Can you work these out from the model? Positions are in its coordinate system, mm. Face numbers are marked on the shaded views. A direction names the side the tool comes from. Give positions to 0.01 mm unless a question says otherwise; leave off trailing zeros. Order: outer loops, then holes, each group sorted by start corner. A loop starts at its lowest first (then second) coordinate and runs counter-clockwise, first axis right, second up. Notation, with made-up numbers: (13.25, 28) - (38.25, 28) arc R16 cw to (38.25, 47) - close; hole circle Ø7 at (76, 35.25). An arc over 180 degrees is marked (long way). Return JSON: item names as keys, results as strings.
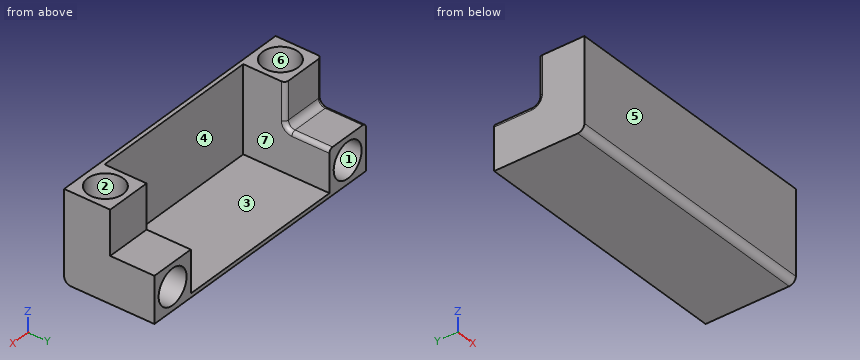
```python
from build123d import *

# Parameters (mm, degrees)
SKETCH1_R           = 13.2
BOSS_EXTRUDE3_DEPTH = 5
SKETCH1_6_W         = 100
SKETCH1_6_H         = 55
SKETCH1_6_R         = 13.2
BOSS_EXTRUDE4_DEPTH = 55
SKETCH2_W           = 65.6
SKETCH2_H           = 52
CUT_EXTRUDE1_DEPTH  = 52
SKETCH3_R           = 13.2
CUT_EXTRUDE2_DEPTH  = 22.6
SKETCH4_W           = 20.6
SKETCH4_H           = 20.6
CUT_EXTRUDE4_DEPTH  = 39
SKETCH9_R           = 13.2
BOSS_EXTRUDE5_DEPTH = 12.4
BOSS_EXTRUDE7_START = 12.4
SKETCH10_R          = 13.2
BOSS_EXTRUDE7_DEPTH = 12.4
MIRROR1_START       = 30.398461356
MIRROR1_OUTLINE_R   = 13.2
MIRROR1_DEPTH       = 37.001538644
MIRROR1_2_OUTLINE_W = 100
MIRROR1_2_OUTLINE_H = 67.4
MIRROR1_2_OUTLINE_R = 13.2
MIRROR1_2_DEPTH     = 3
MIRROR1_3_OUTLINE_W = 34.4
MIRROR1_3_OUTLINE_H = 33
MIRROR1_3_DEPTH     = 4.001538644
MIRROR1_START_2     = 3
MIRROR1_4_OUTLINE_R = 13.2
MIRROR1_4_DEPTH     = 0.998461256
MIRROR1_START_3     = 3.998461256
MIRROR1_5_OUTLINE_R = 13.2
MIRROR1_5_DEPTH     = 26.4000001
MIRROR1_START_4     = 4.9
MIRROR1_6_OUTLINE_R = 13.2
MIRROR1_6_DEPTH     = 35
FILLET3_R           = 5
FILLET4_R           = 5
FILLET5_R           = 3
FILLET6_R           = 3


with BuildPart() as part:
    # Sketch1 → Boss-Extrude3 (new body)
    with BuildSketch(Plane(origin=(0, 0, 0), x_dir=(1, 0, 0), z_dir=(0, 1, 0))):
        with Locations(Location((-32.8, 10.3, 0), (0, 0, 270))):
            Circle(SKETCH1_R)
    boss_extrude3 = extrude(amount=BOSS_EXTRUDE3_DEPTH)

    # Sketch1<6> → Boss-Extrude4 (add)
    with BuildSketch(Plane(origin=(0, 0, 0), x_dir=(1, 0, 0), z_dir=(0, 1, 0))):
        Rectangle(SKETCH1_6_W, SKETCH1_6_H)
        with Locations(Location((-32.8, 10.3, 0), (0, 0, 270))):
            Circle(SKETCH1_6_R, mode=Mode.SUBTRACT)
    extrude(amount=BOSS_EXTRUDE4_DEPTH)

    # Sketch2 → Cut-Extrude1 (cut)
    with BuildSketch(Plane(origin=(0, 55, 0), x_dir=(1, 0, 0), z_dir=(0, 1, 0))):
        with Locations((17.2, -1.5)):
            Rectangle(SKETCH2_W, SKETCH2_H)
    extrude(amount=-CUT_EXTRUDE1_DEPTH, mode=Mode.SUBTRACT)

    # Sketch3 → Cut-Extrude2 (cut)
    with BuildSketch(Plane.XY.offset(27.5)):
        with Locations((-32.801538644, 17.198461356)):
            Circle(SKETCH3_R)
    extrude(amount=-CUT_EXTRUDE2_DEPTH, mode=Mode.SUBTRACT)

    # Sketch4 → Cut-Extrude4 (cut)
    with BuildSketch(Plane.ZY.offset(50)):
        with Locations((17.2, 44.7)):
            Rectangle(SKETCH4_W, SKETCH4_H)
    extrude(amount=-CUT_EXTRUDE4_DEPTH, mode=Mode.SUBTRACT)

    # Sketch9 → Boss-Extrude5 (add)
    with BuildSketch(Plane(origin=(0, 55, 0), x_dir=(1, 0, 0), z_dir=(0, 1, 0))):
        Polygon((-50, -6.9), (-15.6, -6.9), (-15.6, 24.5), (50, 24.5), (50, 27.5), (-50, 27.5), align=None)
        with Locations(Location((-32.8, 10.3, 0), (0, 0, 270))):
            Circle(SKETCH9_R, mode=Mode.SUBTRACT)
    extrude(amount=BOSS_EXTRUDE5_DEPTH)

    # Sketch10 → Boss-Extrude7 (add)
    with BuildSketch(Plane.XY.offset(27.5).offset(BOSS_EXTRUDE7_START)):
        Polygon((-15.6, 3), (-15.6, 34.4), (-50, 34.4), (-50, 0), (50, 0), (50, 3), align=None)
        with Locations((-32.801538644, 17.198461356)):
            Circle(SKETCH10_R, mode=Mode.SUBTRACT)
    extrude(amount=-BOSS_EXTRUDE7_DEPTH)

    # Mirror1: read off the stored shape, not the designer's step
    # Mirror1 outline → Mirror1 (add)
    with BuildSketch(Plane(origin=(0, 0, 0), x_dir=(1, 0, 0), z_dir=(0, 1, 0)).offset(MIRROR1_START)):
        Polygon((150, -6.9), (150, 27.5), (50, 27.5), (50, 24.5), (115.6, 24.5), (115.6, -6.9), align=None)
        with Locations((132.8, 10.3)):
            Circle(MIRROR1_OUTLINE_R, mode=Mode.SUBTRACT)
    extrude(amount=MIRROR1_DEPTH)

    # Mirror1 2 outline → Mirror1 2 (add)
    with BuildSketch(Plane(origin=(0, 0, 0), x_dir=(1, 0, 0), z_dir=(0, 1, 0))):
        with Locations((100, -6.2)):
            Rectangle(MIRROR1_2_OUTLINE_W, MIRROR1_2_OUTLINE_H)
        with Locations((132.8, 10.3)):
            Circle(MIRROR1_2_OUTLINE_R, mode=Mode.SUBTRACT)
    extrude(amount=MIRROR1_2_DEPTH)

    # Mirror1 3 outline → Mirror1 3 (add)
    with BuildSketch(Plane(origin=(0, 0, 0), x_dir=(1, 0, 0), z_dir=(0, 1, 0)).offset(MIRROR1_START)):
        with Locations((132.8, -23.4)):
            Rectangle(MIRROR1_3_OUTLINE_W, MIRROR1_3_OUTLINE_H)
    extrude(amount=MIRROR1_3_DEPTH)

    # Mirror1 4 outline → Mirror1 4 (add)
    with BuildSketch(Plane(origin=(0, 0, 0), x_dir=(1, 0, 0), z_dir=(0, 1, 0)).offset(MIRROR1_START_2)):
        Polygon((150, 27.5), (50, 27.5), (50, 24.5), (115.6, 24.5), (115.6, -39.9), (150, -39.9), align=None)
        with Locations((132.8, 10.3)):
            Circle(MIRROR1_4_OUTLINE_R, mode=Mode.SUBTRACT)
    extrude(amount=MIRROR1_4_DEPTH)

    # Mirror1 5 outline → Mirror1 5 (add)
    with BuildSketch(Plane(origin=(0, 0, 0), x_dir=(1, 0, 0), z_dir=(0, 1, 0)).offset(MIRROR1_START_3)):
        Polygon((150, -39.9), (150, 27.5), (50, 27.5), (50, 24.5), (115.6, 24.5), (115.6, -39.9), align=None)
        with Locations((132.8, 10.3)):
            Circle(MIRROR1_5_OUTLINE_R, mode=Mode.SUBTRACT)
    extrude(amount=MIRROR1_5_DEPTH)

    # Mirror1 6 outline → Mirror1 6 (cut)
    with BuildSketch(Plane.XY.offset(MIRROR1_START_4)):
        with Locations((132.801538644, 17.198461356)):
            Circle(MIRROR1_6_OUTLINE_R)
    extrude(amount=MIRROR1_6_DEPTH, mode=Mode.SUBTRACT)

    # Mirror2: Boss-Extrude3 across plane
    add(boss_extrude3.mirror(Plane.ZY.offset(-50)))

    # Fillet3
    fillet3_edges = [part.edges().sort_by_distance(p)[0] for p in [
        (50, 0, -27.5),
    ]]
    fillet(fillet3_edges, radius=FILLET3_R)

    # Fillet4
    fillet4_edges = [part.edges().sort_by_distance(p)[0] for p in [
        (-32.8, 34.4, 6.9),
    ]]
    fillet(fillet4_edges, radius=FILLET4_R)

    # Fillet5
    fillet5_edges = [part.edges().sort_by_distance(p)[0] for p in [
        (-50, 34.4, 25.9),
        (-50, 35.864466094, 8.364466094),
        (-50, 53.4, 6.9),
    ]]
    fillet(fillet5_edges, radius=FILLET5_R)

    # Fillet6
    fillet6_edges = [part.edges().sort_by_distance(p)[0] for p in [
        (-15.6, 34.4, 25.9),
        (-15.6, 35.864466094, 8.364466094),
        (-15.6, 53.4, 6.9),
    ]]
    fillet(fillet6_edges, radius=FILLET6_R)


solid = part.part
```
1. Suppose I cut it at A-A (y = 56.5). List the corners of the cut face in (x, z) for me.
Checks:
{"outline": "(-50, -27.5) - (150, -27.5) - (150, 6.9) - (115.6, 6.9) - (115.6, -24.5) - (-15.6, -24.5) - (-15.6, 3.9) arc R3 ccw to (-18.6, 6.9) - (-47, 6.9) arc R3 ccw to (-50, 3.9) - close; hole circle Ø26.4 at (-32.8, -10.3); hole circle Ø26.4 at (132.8, -10.3)"}
2. For pin 1 Ø2 at (x, y) = (22.5, 16.5) entering from +Z; pin 2 Ø14 at (x, y) = (-35, 59.5) entering from +Z; pin 3 Ø10 at (x, z) = (140, 17) entering from +Y, each with a flat end and sliding along its axis, tell me the tip position at first contact or that it passes through.
Checks:
{"pin 1": "z = -24.5", "pin 2": "z = 6.9", "pin 3": "y = 34.4"}
3. Suppose I cut it at D-D (z = 35.5). List the corners of the cut face in (x, y) for me, plus the area to 3 significant figures.
Checks:
{"outline": "(-50, 0) - (150, 0) - (150, 34.4) - (115.6, 34.4) - (115.6, 3) - (-15.6, 3) - (-15.6, 31.4) arc R3 ccw to (-18.6, 34.4) - (-47, 34.4) arc R3 ccw to (-50, 31.4) - close; hole circle Ø26.4 at (-32.8, 17.2); hole circle Ø26.4 at (132.8, 17.2)", "area": "1,660 mm^2"}
4. On a 3-axis mill with a long thin cutter (end or side, diameter ignored), from which of +Z, -Z, +X, -X, +Y, -Y can I reach the whole of each face in a straight line? I mean the marked faces 1, 2 and 3. Say none if no direction works.
Checks:
{"face 1": "+Y", "face 2": "+Z", "face 3": "+Z, +Y"}
5. Suppose I cut it at B-B (x = -32.8). List the corners of the cut face in (y, z) for me.
Checks:
{"outline": "(0, -22.5) arc R5 ccw to (5, -27.5) - (67.4, -27.5) - (67.4, -23.5) - (5, -23.5) - (5, 2.9) - (67.4, 2.9) - (67.4, 6.9) - (39.4, 6.9) arc R5 cw to (34.4, 11.9) - (34.4, 39.9) - (30.4, 39.9) - (30.4, 4.9) - (4, 4.9) - (4, 39.9) - (0, 39.9) - close"}
6. Suppose I cut it at C-C (z = -10.3). List the corners of the cut face in (x, y) for me.
Checks:
{"outline": "(-50, 0) - (150, 0) - (150, 67.4) - (146, 67.4) - (146, 5) - (119.6, 5) - (119.6, 67.4) - (115.6, 67.4) - (115.6, 3) - (-15.6, 3) - (-15.6, 67.4) - (-19.6, 67.4) - (-19.6, 5) - (-46, 5) - (-46, 67.4) - (-50, 67.4) - close"}
7. If I drill on L1, parallel to X at y = 28, z = -10.3; L2, parallel to Z at x = -32, y = 49; L3, parallel to X at y = 54.5, z = -3.5, over which ranges is the centre line in solid material (lowest first)? Write a range as [from, to].
Checks:
{"L1": "[-50, -46], [-19.6, -15.6], [115.6, 119.6], [146, 150]", "L2": "[-27.5, -23.48], [2.88, 6.9]", "L3": "[-50, -44.11], [-21.49, -15.6], [115.6, 121.49], [144.11, 150]"}
8. Thinking about a two-plate mould opening in Y: for the marked faces 4, 5, 6 and 7, which applies, +Y half, -Y half, draft (parallel to the pull), parting line (faces both ways), or undercut?
Checks:
{"face 4": "+Y half", "face 5": "-Y half", "face 6": "undercut", "face 7": "draft"}
